Verification items for the finished model (mm, model axes). Coordinates: 2 decimals unless noted, no trailing zeros. Loops run counter-clockwise (first coordinate to the right, second up) from the corner with the lowest first, then second, coordinate; pieces in that order, holes last. Notation, with made-up numbers: (70, -3) -> (115, -3) arc R14 ccw to (115, 1) -> close; hole circle Ø2 at (18, -25). An arc over 180 degrees is marked (long way). Use CSV: the item, a comma, the result in double quotes. Start each with the question number.
```python
from build123d import *

# Parameters (mm, degrees)
SKETCH1_W                                           = 120
SKETCH1_H                                           = 80
BOSS_EXTRUDE1_DEPTH                                 = 1.6
CSK_FOR_M3_COUNTERSUNK_FLAT_HEAD_SCREW1_D           = 3.4
CSK_FOR_M3_COUNTERSUNK_FLAT_HEAD_SCREW1_DEPTH       = 30
CSK_FOR_M3_COUNTERSUNK_FLAT_HEAD_SCREW1_CSINK_D     = 6.3
CSK_FOR_M3_COUNTERSUNK_FLAT_HEAD_SCREW1_CSINK_ANGLE = 90
CSK_FOR_M3_COUNTERSUNK_FLAT_HEAD_SCREW1_TIP         = 1.021463052


with BuildPart() as part:
    # Sketch1 → Boss-Extrude1 (new body)
    with BuildSketch(Plane(origin=(0, 0, 0), x_dir=(1, 0, 0), z_dir=(0, 1, 0))):
        with Locations((60, 40)):
            Rectangle(SKETCH1_W, SKETCH1_H)
    extrude(amount=BOSS_EXTRUDE1_DEPTH)

    # CSK for M3 Countersunk Flat Head Screw1
    with Locations(Plane(origin=(0, 1.6, 0), x_dir=(1, 0, 0), z_dir=(0, 1, 0))):
        with Locations((5, 75), (5, 5), (115, 5), (115, 75)):
            CounterSinkHole(CSK_FOR_M3_COUNTERSUNK_FLAT_HEAD_SCREW1_D / 2, CSK_FOR_M3_COUNTERSUNK_FLAT_HEAD_SCREW1_CSINK_D / 2, depth=CSK_FOR_M3_COUNTERSUNK_FLAT_HEAD_SCREW1_DEPTH, counter_sink_angle=CSK_FOR_M3_COUNTERSUNK_FLAT_HEAD_SCREW1_CSINK_ANGLE)
            with Locations((0, 0, -(CSK_FOR_M3_COUNTERSUNK_FLAT_HEAD_SCREW1_DEPTH + CSK_FOR_M3_COUNTERSUNK_FLAT_HEAD_SCREW1_TIP / 2))):  # 118° drill point
                Cone(0, CSK_FOR_M3_COUNTERSUNK_FLAT_HEAD_SCREW1_D / 2, CSK_FOR_M3_COUNTERSUNK_FLAT_HEAD_SCREW1_TIP, mode=Mode.SUBTRACT)


solid = part.part
```
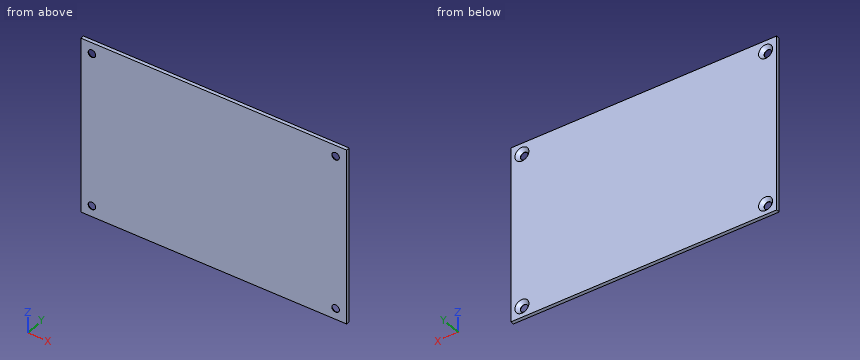
1. Scan lines: line 1 (X direction, y = 0.1, z = -5); line 2 (Z direction, x = 115, y = 0.15); line 3 (Z direction, x = 113.5, y = 0.25). Record each from-to range of solid material in increasing order.
2. Cross-section at A-A, the plane z = -5. Record the boundary of the cut face in (x, y).
3. Cross-section at B-B, the plane x = 5. Record the boundary of the cut face in (y, z).
Solution:
1,line 1,"x = 0 to 3.3, 6.7 to 113.3, 116.7 to 120"
1,line 2,"z = -80 to -76.7, -73.3 to -6.7, -3.3 to 0"
1,line 3,"z = -80 to -75.99, -74.01 to -5.99, -4.01 to 0"
2,outline,"(0, 0) -> (3.3, 0) -> (3.3, 0.15) -> (1.85, 1.6) -> (0, 1.6) -> close; (6.7, 0) -> (113.3, 0) -> (113.3, 0.15) -> (111.85, 1.6) -> (8.15, 1.6) -> (6.7, 0.15) -> close; (116.7, 0) -> (120, 0) -> (120, 1.6) -> (118.15, 1.6) -> (116.7, 0.15) -> close"
3,outline,"(0, -80) -> (1.6, -80) -> (1.6, -78.15) -> (0.15, -76.7) -> (0, -76.7) -> close; (0, -73.3) -> (0.15, -73.3) -> (1.6, -71.85) -> (1.6, -8.15) -> (0.15, -6.7) -> (0, -6.7) -> close; (0, -3.3) -> (0.15, -3.3) -> (1.6, -1.85) -> (1.6, 0) -> (0, 0) -> close"
